from build123d import *

# Parameters (mm, degrees)
SKETCH006_R   = 39.497
PAD001_DEPTH  = 6.096
SKETCH007_R   = 57.9374
SKETCH007_R_2 = 1.8034
PAD002_DEPTH  = 2.032
SKETCH009_R   = 36.957
POCKET_DEPTH  = 5.08


with BuildPart() as part:
    # Sketch006 → Pad001 (new body)
    with BuildSketch(Plane.XY):
        with Locations((177.8, 177.8)):
            Circle(SKETCH006_R)
    extrude(amount=PAD001_DEPTH)

    # Sketch007 → Pad002 (join)
    with BuildSketch(Plane.XY):
        with Locations((177.8, 177.8)):
            Circle(SKETCH007_R)
        with Locations((220.210303, 202.2856)):
            Circle(SKETCH007_R_2, mode=Mode.SUBTRACT)
        with Locations((135.389697, 202.2856)):
            Circle(SKETCH007_R_2, mode=Mode.SUBTRACT)
        with Locations((177.8, 128.8288)):
            Circle(SKETCH007_R_2, mode=Mode.SUBTRACT)
    extrude(amount=-PAD002_DEPTH)

    # Sketch009 (on Face3 of Pad002) → Pocket (cut)
    with BuildSketch(Plane(origin=(0, 0, -2.032), x_dir=(1, 0, 0), z_dir=(0, 0, -1))):
        with Locations((177.8, -177.8)):
            Circle(SKETCH009_R)
    extrude(amount=-POCKET_DEPTH, mode=Mode.SUBTRACT)


solid = part.part
Design review of the part built by this model. Coordinates are the model's own, in mm. A direction names the side the tool comes from. Round coordinates to 2 decimals unless told otherwise and drop trailing zeros. Write each loop counter-clockwise with the first axis right and the second up, starting at its lowest first coordinate (ties: lowest second). Pieces come first, ordered by that corner, then holes. Notation, with made-up numbers: (85.5, 52) -> (131.5, 52) arc R28 ccw to (131.5, 82) -> close; hole circle Ø1 at (32, 8.5). An arc over 180 degrees is marked (long way). One line per question, with ' | ' between items.
(1) Take a section at C-C, the plane x = 158. State the section outline as (y, z) points, and give its area (3 significant figures).
Result sheet:
outline: (123.35, -2.03) -> (146.59, -2.03) -> (146.59, 3.05) -> (209.01, 3.05) -> (209.01, -2.03) -> (232.25, -2.03) -> (232.25, 0) -> (211.98, 0) -> (211.98, 6.1) -> (143.62, 6.1) -> (143.62, 0) -> (123.35, 0) -> close | area: 321 mm2
(2) Take a section at A-A, the plane x = 177.8. State the section outline as (y, z) points.
Result sheet:
outline: (119.86, -2.03) -> (127.03, -2.03) -> (127.03, 0) -> (119.86, 0) -> close; (130.63, -2.03) -> (140.84, -2.03) -> (140.84, 3.05) -> (214.76, 3.05) -> (214.76, -2.03) -> (235.74, -2.03) -> (235.74, 0) -> (217.3, 0) -> (217.3, 6.1) -> (138.3, 6.1) -> (138.3, 0) -> (130.63, 0) -> close
(3) Take a section at B-B, the plane y = 177.8. State the section outline as (x, z) points.
Result sheet:
outline: (119.86, -2.03) -> (140.84, -2.03) -> (140.84, 3.05) -> (214.76, 3.05) -> (214.76, -2.03) -> (235.74, -2.03) -> (235.74, 0) -> (217.3, 0) -> (217.3, 6.1) -> (138.3, 6.1) -> (138.3, 0) -> (119.86, 0) -> close
(4) Machinability: for faces 4 (the flat face through (190, 140, 0)), 5 (the flat face through (177, 177, 3.048)), 6 (the cylindrical face through (218.41, 202.36, -1)), which of the approach directions +Z, -Z, +X, -X, +Y, -Y give a long, thin tool a straight path to every point of the face, cutting with its end or side? Answer none if there is none.
Result sheet:
face 4: +Z | face 5: -Z | face 6: +Z, -Z
(5) Draft analysis for pull direction X (two halves, no side actions). For faces 1 (the flat face through (177, 140, -2.032)), 2 (the cylindrical face through (215.473, 189.664, 3.005)), 3 (the cylindrical face through (148.472, 200.288, 0.472)), state which applies: released by +X, released by -X, zero draft, split by the parting line, or undercut.
Result sheet:
face 1: zero draft | face 2: split by the parting line | face 3: undercut
(6) Wall thickness on line 1 (Y direction, x = 177.8, z = 0.3); line 2 (X direction, y = 178.5, z = 2): over which ranges is each line inside the solid? List them lowest first. Write a range as [from, to].
Result sheet:
line 1: [138.3, 140.84], [214.76, 217.3] | line 2: [138.31, 140.85], [214.75, 217.29]
(7) Take a section at D-D, the plane y = 225.5. State the section outline as (x, z) points, and give its area (3 significant figures).
Result sheet:
outline: (144.91, -2.03) -> (210.69, -2.03) -> (210.69, 0) -> (144.91, 0) -> close | area: 134 mm2
(8) Insertion check: P1, Ø1, axis at x = 181, y = 162, coming from the -Z side; P2, Ø3, axis at y = 187.5, z = 5, coming from the +X side; P3, Ø4, axis at y = 149, z = -1, coming from the +X side. Each pin has a flat end and moves straight along its axis. Give the tip position at first contact, or say it passes through.
Result sheet:
P1: z = 3.05 | P2: x = 216.44 | P3: x = 229.17
